For this review, take the finished solid that the model builds, in its own axes (mm). A direction names the side the tool comes from. Round coordinates to 2 decimals unless told otherwise and drop trailing zeros. Write each loop counter-clockwise with the first axis right and the second up, starting at its lowest first coordinate (ties: lowest second). Pieces come first, ordered by that corner, then holes. Notation, with made-up numbers: (72, 67.25) -> (124, 67.25) arc R23 ccw to (124, 94.25) -> close; hole circle Ø4 at (80, 81). An arc over 180 degrees is marked (long way). Answer in a Markdown table with one row per item.
Autodesk Inventor part; units mm, degrees
ref_plane "Work Plane1" through (230, 25, 3) normal (0, 0.7071068, 0.7071068) x (1, 0, 0)
ref_plane "YZ Plane" through (0, 0, 0) normal (1, 0, 0) x (0, 1, 0)
ref_plane "XZ Plane" through (0, 0, 0) normal (0, 1, 0) x (-1, 0, 0)
sketch "Sketch3" plane through (230, 25, 3) normal (0, 0.7071068, 0.7071068) x (1, 0, 0)
  line L0 (0, 0) -> (-460, 0)
  line L1 (-460, 0) -> (-460, 27.12132)
  line L2 (-460, 27.12132) -> (0, 27.12132)
  line L3 (0, 27.12132) -> (0, 0)
  line L4 (0, 2.12132) -> (-460, 2.12132)
  line L5 (-460, -35.355339) -> (-460, 0)
  point P0 (-230, -15.556349)
  dimension "d4" = 25
  dimension "d5" = 0
sketch "Sketch1 outline for Plate1" plane through (0, 0, 0) normal (0, 0, 1) x (1, 0, 0)
  line L0 (-230, 25) -> (-230, -25)
  line L1 (230, 25) -> (-230, 25)
  line L2 (230, -25) -> (230, 25)
  line L3 (-230, -25) -> (230, -25)
extrude "Plate1" add sketch "Sketch1 outline for Plate1" along normal blind 3
sketch "Sketch1" plane through (0, 0, 0) normal (0, 0, 1) x (1, 0, 0)
  line L0 (-230, -25) -> (230, -25)
  line L1 (230, -25) -> (230, 25)
  line L2 (230, 25) -> (-230, 25)
  line L3 (-230, 25) -> (-230, -25)
  line L4 (-230, -25) -> (230, 25) construction
  line L5 (230, -25) -> (-230, 25) construction
  point P0 (0, 0)
  dimension "d0" = 460
  dimension "d1" = 50
ref_plane "Work Plane1" through (230, 25, 3) normal (0, 0.7071068, 0.7071068) x (1, 0, 0)
sketch "Sketch3 outline for Plate2" plane through (230, 25, 3) normal (0, 0.7071068, 0.7071068) x (1, 0, 0)
  line L0 (0, 0) -> (-460, 0)
  line L1 (-460, 0) -> (-460, 27.12132)
  line L2 (-460, 27.12132) -> (0, 27.12132)
  line L3 (0, 27.12132) -> (0, 2.12132)
  line L4 (0, 2.12132) -> (0, 0)
sheet face with bend "Face2" sketch "Sketch3 outline for Plate2" thickness 3 toward (0, -0.7071068, -0.7071068) bend radius 3
bend "Bend1"
equation "\"d2\" = Thickness"
equation "\"d6\" = BendRadius"
equation "\"d7\" = BendReliefWidth"
equation "\"d9\" = MinimumRemnant"
equation "\"d8\" = BendReliefDepth"
equation "\"d10\" = TransitionRadius"
equation "\"BendRadius\" = Thickness"
equation "\"BendReliefWidth\" = Thickness"
equation "\"BendReliefDepth\" = 0.5 * Thickness"
equation "\"CornerReliefSize\" = 4 * Thickness"
equation "\"MinimumRemnant\" = 2 * Thickness"
equation "\"TransitionRadius\" = BendRadius"
equation "\"JacobiRadiusSize\" = BendRadius"
equation "\"GapSize\" = Thickness"
properties part number "Skena"
1) Consider section B-B on y = -1. State the section outline as (x, z) points.
Solved:
| item | result |
|---|---|
| outline | (-230, 0) -> (230, 0) -> (230, 3) -> (-230, 3) -> close |
2) Consider section C-C on z = -12.25. State the section outline as (x, y) points, then the cut area to 3 significant figures.
Solved:
| item | result |
|---|---|
| outline | (-230, 36.01) -> (230, 36.01) -> (230, 40.25) -> (-230, 40.25) -> close |
| area | 1,950 mm² |
3) For faces 1 (the flat face through (-3, 36, -8)), 2 (the flat face through (-3, -1, 0)), list the 3-axis set-ups (+Z, -Z, +X, -X, +Y, -Y) from which the entire face can be reached by the end or side of a thin tool; tool diameter is ignored.
Solved:
| item | result |
|---|---|
| face 1 | +Z, +X, -X, +Y |
| face 2 | -Z, +X, -X, -Y |
4) Clearance check with flat-ended pins moving along their axes: pin 1 Ø5 at (x, y) = (54.5, 34) entering from +Z; pin 2 Ø3 at (x, z) = (97, -4.5) entering from -Y; pin 3 Ø3 at (x, y) = (155.5, 37) entering from +Z. State where each tip first meets the part, or that it passes through.
Solved:
| item | result |
|---|---|
| pin 1 | z = -3.5 |
| pin 2 | y = 26.76 |
| pin 3 | z = -7.5 |
5) For line 1 (Z direction, x = -123.5, y = 12.5); line 2 (Y direction, x = 161.5, z = -4.75); line 3 (Y direction, x = 94.5, z = 1), list the stretches that pass through material, from the lowest coordinate up. Write a range as [from, to].
Solved:
| item | result |
|---|---|
| line 1 | [0, 3] |
| line 2 | [28.51, 32.75] |
| line 3 | [-25, 27] |
6) Consider section A-A on x = -123. State the section outline as (y, z) points.
Solved:
| item | result |
|---|---|
| outline | (-25, 0) -> (22.51, 0) arc R3 cw to (24.64, -0.88) -> (42.06, -18.3) -> (44.18, -16.18) -> (26.76, 1.24) arc R6 ccw to (22.51, 3) -> (-25, 3) -> close |
